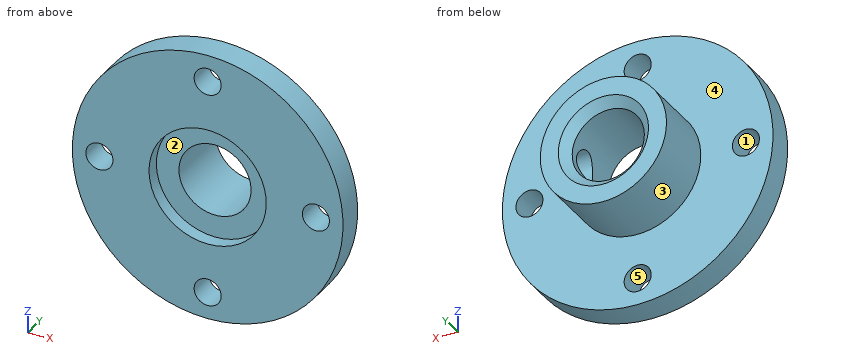
```python
from build123d import *

# Parameters (mm, degrees)
SKETCH_1_R          = 15
SKETCH_1_R_2        = 4
EXTRUDE_1_DEPTH     = 3
SKETCH_2_R          = 7
SKETCH_2_R_2        = 4
EXTRUDE_2_DEPTH     = 7
SKETCH_5_R          = 1.65
CUT_EXTRUDE_1_DEPTH = 12
SKETCH_6_R          = 6.5
CUT_EXTRUDE_2_DEPTH = 1.5
SKETCH_7_R          = 1.5
CUT_EXTRUDE_3_DEPTH = 4
CHAMFER_1_SIZE      = 1


with BuildPart() as part:
    # Sketch 1 → Extrude 1 (new body)
    with BuildSketch(Plane(origin=(0, 0, 0), x_dir=(1, 0, 0), z_dir=(0, 1, 0))):
        with Locations(Location((0, 0, 0), (0, 0, 270))):
            Circle(SKETCH_1_R)
        with Locations(Location((0, 0, 0), (0, 0, 270))):
            Circle(SKETCH_1_R_2, mode=Mode.SUBTRACT)
    extrude(amount=EXTRUDE_1_DEPTH)

    # Sketch 2 → Extrude 2 (add)
    with BuildSketch(Plane(origin=(0, 3, 0), x_dir=(1, 0, 0), z_dir=(0, 1, 0))):
        with Locations(Location((0, 0, 0), (0, 0, 270))):
            Circle(SKETCH_2_R)
        with Locations(Location((0, 0, 0), (0, 0, 270))):
            Circle(SKETCH_2_R_2, mode=Mode.SUBTRACT)
    extrude(amount=EXTRUDE_2_DEPTH)

    # Sketch 5 → Cut-Extrude 1 (cut)
    with BuildSketch(Plane.ZY):
        with Locations((0, 6.5)):
            Circle(SKETCH_5_R)
    extrude(amount=-CUT_EXTRUDE_1_DEPTH, mode=Mode.SUBTRACT)

    # Sketch 6 → Cut-Extrude 2 (cut)
    with BuildSketch(Plane.XZ):
        with Locations(Location((0, 0, 0), (0, 0, 270))):
            Circle(SKETCH_6_R)
    extrude(amount=-CUT_EXTRUDE_2_DEPTH, mode=Mode.SUBTRACT)

    # Sketch 7 → Cut-Extrude 3 (cut)
    with BuildSketch(Plane(origin=(0, 3, 0), x_dir=(1, 0, 0), z_dir=(0, 1, 0))):
        with Locations(Location((12, 0, 0), (0, 0, 270))):
            Circle(SKETCH_7_R)
        with Locations(Location((0, -12, 0), (0, 0, 270))):
            Circle(SKETCH_7_R)
        with Locations(Location((-12, 0, 0), (0, 0, 270))):
            Circle(SKETCH_7_R)
        with Locations(Location((0, 12, 0), (0, 0, 270))):
            Circle(SKETCH_7_R)
    extrude(amount=-CUT_EXTRUDE_3_DEPTH, mode=Mode.SUBTRACT)

    # Chamfer 1
    chamfer_1_edges = [part.edges().sort_by_distance(p)[0] for p in [
        (0, 10, -4),
    ]]
    chamfer(chamfer_1_edges, length=CHAMFER_1_SIZE)


solid = part.part
```
Model file for the job. Use its own axes, mm. Face numbers are marked on the shaded views. A direction names the side the tool comes from. Give positions to 0.01 mm unless a question says otherwise; leave off trailing zeros. Write each loop counter-clockwise with the first axis right and the second up, starting at its lowest first coordinate (ties: lowest second). Pieces come first, ordered by that corner, then holes. Notation, with made-up numbers: M 46.25,-35 L 68.25,-35 A22 ccw 68.25,-15 Z; hole C 29,20 d8. An arc over 180 degrees is marked long. Use a Markdown table: item, result.
1) Tool access for the marked faces 1 and 2: list every direction of +Z, -Z, +X, -X, +Y, -Y with a clear straight run to the whole face (end or side of a thin tool).
Responses:
| item | result |
|---|---|
| face 1 | +Y, -Y |
| face 2 | -Y |
2) Pull direction Z, two halves, no side cores. Call the marked faces 3, 4 and 5: +Z half, -Z half, draft (parallel to the pull), parting line (faces both ways), or undercut.
Responses:
| item | result |
|---|---|
| face 3 | parting line |
| face 4 | draft |
| face 5 | undercut |
3) Cut at C-C (y = 2). List the corners of the cut face in (x, z), and give its area (3 significant figures).
Responses:
| item | result |
|---|---|
| outline | C 0,0 d30; hole C -12,0 d3; hole C 0,0 d8; hole C 0,-12 d3; hole C 0,12 d3; hole C 12,0 d3 |
| area | 628 mm2 |
4) Cut at A-A (x = 12). List the corners of the cut face in (y, z).
Responses:
| item | result |
|---|---|
| outline | M 0,-9 L 3,-9 L 3,-1.5 L 0,-1.5 Z; M 0,1.5 L 3,1.5 L 3,9 L 0,9 Z |
5) Cut at D-D (y = 8.5). List the corners of the cut face in (x, z).
Responses:
| item | result |
|---|---|
| outline | C 0,0 d14; hole C 0,0 d8 |
6) Cut at B-B (z = 12). List the corners of the cut face in (x, y).
Responses:
| item | result |
|---|---|
| outline | M -9,0 L -1.5,0 L -1.5,3 L -9,3 Z; M 1.5,0 L 9,0 L 9,3 L 1.5,3 Z |
7) Drill centre lines: line 1 (Y direction, x = 6.35, z = 0); line 2 (Z direction, x = -1, y = 2.5); line 3 (Y direction, x = -2.5, z = -7.25). Where is each one in solid material? Low to high. Write a range as from..to.
Responses:
| item | result |
|---|---|
| line 1 | y = 1.5..4.85, 8.15..10 |
| line 2 | z = -14.97..-13.12, -10.88..-3.87, 3.87..10.88, 13.12..14.97 |
| line 3 | y = 0..3 |
8) Pin check, flat tips, straight feed: pin 1 (2.5 mm diameter, centred on x = 12, z = 0, fed in from +Y); pin 2 (1 mm diameter, centred on x = -2.5, y = 7.5, fed in from -Z); pin 3 (6.5 mm diameter, centred on x = 2, z = 2.5, fed in from -Y); pin 4 (6 mm diameter, centred on y = 9, z = 0.5, fed in from -X). Stop position of each tip, or through.
Responses:
| item | result |
|---|---|
| pin 1 | passes through |
| pin 2 | stops at z = -6.71 |
| pin 3 | stops at y = 1.5 |
| pin 4 | stops at x = -7 |
